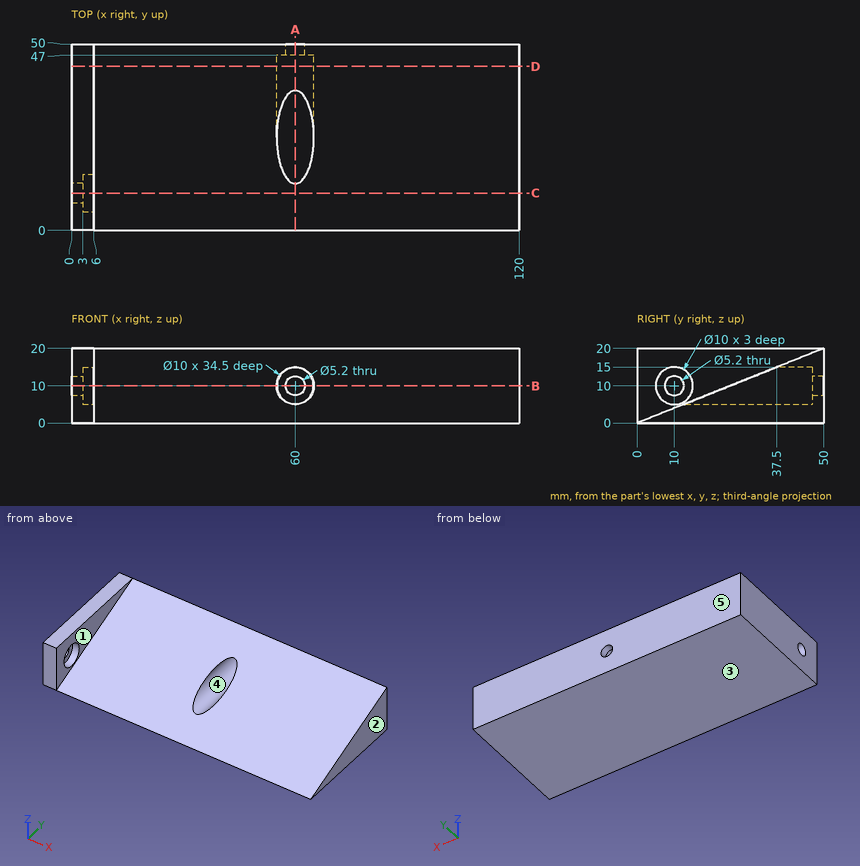
Design review of the part shown in the three views and the two pictorial views. Dimensions are in mm from the part's minimum x, y and z. A direction names the side the tool comes from. Coordinates: 2 decimals unless noted, no trailing zeros. Order: outer loops, then holes, each group sorted by start corner. A loop starts at its lowest first (then second) coordinate and runs counter-clockwise, first axis right, second up.
Item 1: Take a section at D-D, the plane y = 44. Write out the cut boundary in (x, z), then the cut area to 3 significant figures.
Item 2: The part is to be moulded in two halves that separate along Z. For the marked faces 3, 4 and 5, say which applies: pulls with the +Z half, pulls with the -Z half, needs draft (parallel to the pull), parting line crosses it, or undercut.
Item 3: Take a section at C-C, the plane y = 10. Write out the cut boundary in (x, z).
Item 4: Take a section at A-A, the plane x = 60. Write out the cut boundary in (y, z).
Item 5: For pin 1 Ø3 at (x, z) = (60, 10) entering from +Y; pin 2 Ø8.5 at (y, z) = (10, 10) entering from -X; pin 3 Ø10 at (x, y) = (27, 16.5) entering from +Z; pin 4 Ø8 at (y, z) = (11.5, 12) entering from +X, all flat-tipped, find the tip position at first contact; note any pin that passes through.
Item 6: For the marked faces 1 and 2, list the 3-axis set-ups (+Z, -Z, +X, -X, +Y, -Y) from which the entire face can be reached by the end or side of a thin tool; tool diameter is ignored.
Item 7: Take a section at B-B, the plane z = 10. Write out the cut boundary in (x, y).
Item 8: For line 1 (X direction, y = 30, z = 10); line 2 (Z direction, x = 1.25, y = 10); line 3 (X direction, y = 12, z = 5.5), list the stretches that pass through material, from the lowest coordinate up.
The answers:
1. outline: (0, 0) - (120, 0) - (120, 17.6) - (6, 17.6) - (6, 20) - (0, 20) - close; hole circle Ø10 at (60, 10)
1. area: 2,050 mm2
2. face 3: pulls with the -Z half
2. face 4: undercut
2. face 5: needs draft
3. outline: (0, 0) - (120, 0) - (120, 4) - (6, 4) - (6, 5) - (3, 5) - (3, 7.4) - (0, 7.4) - close; (0, 12.6) - (3, 12.6) - (3, 15) - (6, 15) - (6, 20) - (0, 20) - close
4. outline: (0, 0) - (50, 0) - (50, 7.4) - (47, 7.4) - (47, 5) - (12.5, 5) - close; (37.5, 15) - (47, 15) - (47, 12.6) - (50, 12.6) - (50, 20) - close
5. pin 1: passes through
5. pin 2: stops at x = 0
5. pin 3: stops at z = 8.6
5. pin 4: stops at x = 6
6. face 1: +Z, +X, -Y
6. face 2: +Z, -Z, +X, +Y, -Y
7. outline: (0, 0) - (6, 0) - (6, 5) - (3, 5) - (3, 7.4) - (0, 7.4) - close; (0, 12.6) - (3, 12.6) - (3, 15) - (6, 15) - (6, 25) - (55, 25) - (55, 47) - (57.4, 47) - (57.4, 50) - (0, 50) - close; (62.6, 47) - (65, 47) - (65, 25) - (120, 25) - (120, 50) - (62.6, 50) - close
8. line 1: x = 0 to 55, 65 to 120
8. line 2: z = 0 to 7.4, 12.6 to 20
8. line 3: x = 0 to 3
